```python
from build123d import *

# Parameters (mm, degrees)
SKETCH_1_R               = 30
EXTRUDE_1_DEPTH          = 3
SKETCH_2_W               = 11
SKETCH_2_H               = 11
EXTRUDE_2_DEPTH          = 4
SKETCH_4_R               = 6
CUT_EXTRUDE_1_DEPTH      = 25
SKETCH_5_R               = 9
CUT_EXTRUDE_2_DEPTH      = 9
CUT_EXTRUDE_START        = 7.85
SKETCH_6_R               = 10
SKETCH_6_R_2             = 9
CUT_EXTRUDE_3_DEPTH      = 1.1
SKETCH_8_R               = 26.5
EXTRUDE_3_DEPTH          = 5
CUT_EXTRUDE_4_DEPTH      = 88.669835177
CUT_EXTRUDE_4_DEPTH_BACK = 88.669835177
SKETCH_7_R               = 15
SKETCH_10_R              = 2.25
CUT_EXTRUDE_5_DEPTH      = 17


with BuildPart() as part:
    # Sketch 1 → Extrude 1 (new body)
    with BuildSketch(Plane.XY):
        Circle(SKETCH_1_R)
    extrude(amount=EXTRUDE_1_DEPTH)



with BuildPart() as body_2:
    # Sketch 2 → Revolve 1 (revolve)
    with BuildSketch(Plane.XY.offset(3), mode=Mode.PRIVATE) as revolve_1_sk:
        with Locations((64.5, -0.125)):
            Rectangle(SKETCH_2_W, SKETCH_2_H)
    revolve(revolve_1_sk.sketch.rotate(Axis((70, 22.717290725, 3), (0, -1, 0)), 270), axis=Axis((70, 22.717290725, 3), (0, -1, 0)))


with BuildPart() as part_1:
    add(part.part)

    add(body_2.part)  # Extrude 2 merges body 2
    # Sketch 3 → Extrude 2 (add, symmetric)
    with BuildSketch(Plane.XY.offset(3)):
        with BuildLine():
            Line((11.937553945, 27.522623527), (63, 5.375))
            Line((63, 5.375), (63, -4))
            Line((63, -4), (12.555800964, -27.246134811))
            ThreePointArc((12.555800964, -27.246134811), (-29.998088792, -0.338627888), (11.937553945, 27.522623527))
        make_face()
    extrude(amount=EXTRUDE_2_DEPTH, both=True)

    # Sketch 4 → Cut-Extrude 1 (cut)
    with BuildSketch(Plane.XZ.offset(5.625)):
        with Locations(Location((70, 3, 0), (0, 0, 270))):
            Circle(SKETCH_4_R)
    extrude(amount=-CUT_EXTRUDE_1_DEPTH, mode=Mode.SUBTRACT)

    # Sketch 5 → Cut-Extrude 2 (cut)
    with BuildSketch(Plane.XZ.offset(5.625)):
        with Locations(Location((70, 3, 0), (0, 0, 270))):
            Circle(SKETCH_5_R)
    extrude(amount=-CUT_EXTRUDE_2_DEPTH, mode=Mode.SUBTRACT)

    # Sketch 6 → Cut-Extrude 3 (cut)
    # profile 1 of 2: a face of its own
    with BuildSketch(Plane.XZ.offset(-3.375).offset(CUT_EXTRUDE_START)):
        with Locations(Location((70, 3, 0), (0, 0, 270))):
            Circle(SKETCH_6_R)
        with Locations(Location((70, 3, 0), (0, 0, 270))):
            Circle(SKETCH_6_R_2, mode=Mode.SUBTRACT)
    # profile 2 of 2: a face of its own
    with BuildSketch(Plane.XZ.offset(-3.375).offset(CUT_EXTRUDE_START)):
        with Locations(Location((70, 3, 0), (0, 0, 270))):
            Circle(SKETCH_6_R_2)
    extrude(amount=-CUT_EXTRUDE_3_DEPTH, mode=Mode.SUBTRACT)

    # Sketch 8 → Extrude 3 (add, symmetric)
    with BuildSketch(Plane(origin=(0, 0, 3), x_dir=(-1, 0, 0), z_dir=(0, 0, -1))):
        with Locations(Location((0, 0, 0), (0, 0, 180))):
            Circle(SKETCH_8_R)
    extrude(amount=EXTRUDE_3_DEPTH, both=True)

    # Sketch 7 → Cut-Extrude 4 (cut, two sides: drawn at the far end of the back side and taken through both)
    with BuildSketch(Plane.XY.offset(7).offset(-CUT_EXTRUDE_4_DEPTH_BACK)):
        with Locations(Location((0, 0, 0), (0, 0, 180))):
            Circle(SKETCH_7_R)
        with BuildLine():
            Line((26.392321658, -14.26342727), (48.663997023, -4))
            Line((48.663997023, -4), (29.732137495, -4))
            ThreePointArc((29.732137495, -4), (28.527586888, -9.283145284), (26.392321658, -14.26342727))
        make_face()
        with BuildLine():
            Line((29.732137495, 4), (48.663997023, 4))
            Line((48.663997023, 4), (26.392321658, 14.26342727))
            ThreePointArc((26.392321658, 14.26342727), (28.527586888, 9.283145284), (29.732137495, 4))
        make_face()
    extrude(amount=CUT_EXTRUDE_4_DEPTH + CUT_EXTRUDE_4_DEPTH_BACK, mode=Mode.SUBTRACT)

    # Sketch 10 → Cut-Extrude 5 (cut)
    with BuildSketch(Plane.XY.offset(8)):
        with Locations((21.75, 0)):
            Circle(SKETCH_10_R)
        with Locations((13.980630511, -16.661466638)):
            Circle(SKETCH_10_R)
        with Locations(Location((-21.75, 0, 0), (0, 0, 180))):
            Circle(SKETCH_10_R)
        with Locations(Location((-13.980630511, -16.661466638, 0), (0, 0, 180))):
            Circle(SKETCH_10_R)
        with Locations(Location((13.980630511, 16.661466638, 0), (0, 0, 180))):
            Circle(SKETCH_10_R)
        with Locations((-13.980630511, 16.661466638)):
            Circle(SKETCH_10_R)
    extrude(amount=-CUT_EXTRUDE_5_DEPTH, mode=Mode.SUBTRACT)


solid = part_1.part
```
Work out the finished part from the listing and answer in its coordinate system (mm). A direction names the side the tool comes from. Round coordinates to 2 decimals unless told otherwise and drop trailing zeros. Order: outer loops, then holes, each group sorted by start corner. A loop starts at its lowest first (then second) coordinate and runs counter-clockwise, first axis right, second up.
Q1. A cutting plane is placed at C-C, the plane y = -11. Determine the outline of the cut face in (x, z).
Solution:
outline: (-27.91, -1) - (-24.11, -1) - (-24.11, -2) - (-10.2, -2) - (-10.2, 8) - (-24.11, 8) - (-24.11, 7) - (-27.91, 7) - close; (10.2, -2) - (24.11, -2) - (24.11, -1) - (27.91, -1) - (27.91, 7) - (24.11, 7) - (24.11, 8) - (10.2, 8) - close; (33.47, -1) - (47.81, -1) - (47.81, 7) - (33.47, 7) - close
Q2. A cutting plane is placed at B-B, the plane x = 0. Determine the outline of the cut face in (y, z), then the cut area to 3 significant figures.
Solution:
outline: (-30, -1) - (-26.5, -1) - (-26.5, -2) - (-15, -2) - (-15, 8) - (-26.5, 8) - (-26.5, 7) - (-30, 7) - close; (15, -2) - (26.5, -2) - (26.5, -1) - (30, -1) - (30, 7) - (26.5, 7) - (26.5, 8) - (15, 8) - close
area: 286 mm2
Q3. A cutting plane is placed at D-D, the plane z = 1.75. Count the separate pieces of the cut face and the enclosed holes in it, then the cut area to 3 significant figures.
Solution:
separate pieces: 2
enclosed holes: 9
area: 2,780 mm2
Q4. A cutting plane is placed at A-A, the plane y = 0. Determine the outline of the cut face in (x, z).
Solution:
outline: (-30, -1) - (-26.5, -1) - (-26.5, -2) - (-24, -2) - (-24, 8) - (-26.5, 8) - (-26.5, 7) - (-30, 7) - close; (-19.5, -2) - (-15, -2) - (-15, 8) - (-19.5, 8) - close; (15, -2) - (19.5, -2) - (19.5, 8) - (15, 8) - close; (24, -2) - (26.5, -2) - (26.5, -1) - (59.75, -1) arc R11 ccw (long way) to (59.75, 7) - (26.5, 7) - (26.5, 8) - (24, 8) - close; hole circle Ø18 at (70, 3)
Q5. The mould has two halves that part along X. Classify faces 1 (the flat face through (75, 5.375, 8)), 2 (the cylindrical face through (23.896, 0.676, 3.07)), 3 (the cylindrical face through (-29.977, -1.175, 3.056)), 4 (the flat face through (37.111, 16.604, 3.056)): pulls with the +X half, pulls with the -X half, needs draft (parallel to the pull), parting line crosses it, or undercut.
Solution:
face 1: needs draft
face 2: undercut
face 3: parting line crosses it
face 4: pulls with the +X half
Q6. A tool of negligible diameter and unlimited length cuts with its end or side. For faces 5 (the cylindrical face through (61.214, -0.047, 4.951)), 6 (the flat face through (27, 2, -1)), 7 (the flat face through (72, -3.375, 12)), from which of +Z, -Z, +X, -X, +Y, -Y can it reach the whole face along a straight path? Write none if from no direction.
Solution:
face 5: -Y
face 6: -Z
face 7: none
Q7. Find the intervals of material crossed by line 1 along X through (y, z) = (-11, 2.25); line 2 along X through (y, z) = (-6, -0.5); line 3 along Y through (x, z) = (45.5, -0.5), in increasing order.
Solution:
line 1: x = -27.91 to -10.2, 10.2 to 27.91, 33.47 to 47.81
line 2: x = -29.39 to -13.75, 13.75 to 29.39, 44.32 to 58.66
line 3: y = -12.06 to -5.46, -4 to 4, 5.46 to 12.97
Q8. Given pin 1 Ø4 at (y, z) = (-5.5, -5) entering from +X; pin 2 Ø7 at (x, y) = (13.98, 16.66) entering from +Z; pin 3 Ø1 at (x, y) = (40.5, -14) entering from +Z, each flat-ended and moving along its own axis, determine where each tip first touches the part or whether it passes through.
Solution:
pin 1: stops at x = 79.22
pin 2: stops at z = 8
pin 3: stops at z = 7
